Here's how the part is built. I have some questions about the finished solid (model axes, mm). Round coordinates to 2 decimals unless told otherwise and drop trailing zeros. Loops run counter-clockwise (first coordinate to the right, second up) from the corner with the lowest first, then second, coordinate; pieces in that order, holes last. Notation, with made-up numbers: (41, -4.5) - (53, -4.5) arc R21 cw to (53, 32.5) - close; hole circle Ø3 at (22, -6.5). An arc over 180 degrees is marked (long way). Answer as a JSON object with one key per item and string values. Group by question number.
1) I want a section at D-D, the plane x = 110. Please give me the cut outline in (y, z), then the cut area to 3 significant figures.
2) I want a section at A-A, the plane z = -90. Please give me the cut outline in (x, y).
3) Will these pins go through, and if not, where does the flat tip stop? P1, Ø1, axis at x = 47, y = 2, coming from the +Z side; P2, Ø7, axis at x = -110, z = -17.5, coming from the +Y side; P3, Ø10.5, axis at x = 0, z = -127.5, coming from the -Y side.
4) I want a section at B-B, the plane y = 1.65. Please give me the cut outline in (x, z).
5) I want a section at C-C, the plane z = -17.5. Please give me the cut outline in (x, y).
6) If I drill on line 1 along X through (y, z) = (2.95, -80); line 2 along X through (y, z) = (2.95, -17.5); line 3 along Z through (x, y) = (110, 2.85), over which ranges is the centre line in solid material (lowest first)? Write a range as [from, to].
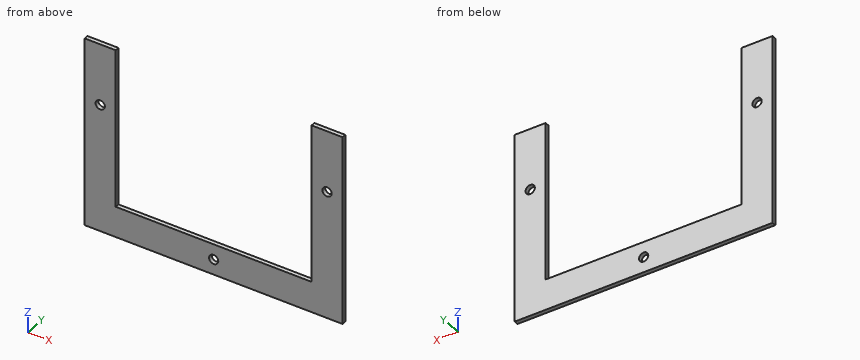
from build123d import *

# Parameters (mm, degrees)
SKETCH1_W            = 250
SKETCH1_H            = 285
SKETCH1_W_2          = 190
SKETCH1_H_2          = 225
EXTRUDE_THIN1_DEPTH  = 4
SKETCH2_W            = 250
SKETCH2_H            = 100
CUT_EXTRUDE1_DEPTH   = 10
SKETCH3_R            = 4.5
CUT_EXTRUDE2_DEPTH   = 10
LPATTERN1_COUNT      = 2
LPATTERN1_PITCH      = 144.5
LPATTERN1_COUNT_DIR2 = 2
LPATTERN1_PITCH_DIR2 = 144.5
SKETCH4_R            = 4.5
CUT_EXTRUDE3_DEPTH   = 10


with BuildPart() as part:
    # Sketch1 → Extrude-Thin1 (new body)
    with BuildSketch(Plane(origin=(0, 0, 0), x_dir=(1, 0, 0), z_dir=(0, 1, 0))):
        Rectangle(SKETCH1_W, SKETCH1_H)
        Rectangle(SKETCH1_W_2, SKETCH1_H_2, mode=Mode.SUBTRACT)
    extrude(amount=EXTRUDE_THIN1_DEPTH)

    # Sketch2 → Cut-Extrude1 (cut)
    with BuildSketch(Plane.XZ):
        with Locations((0, 92.5)):
            Rectangle(SKETCH2_W, SKETCH2_H)
    extrude(amount=-CUT_EXTRUDE1_DEPTH, mode=Mode.SUBTRACT)

    # Sketch3 → Cut-Extrude2 (cut)
    with BuildSketch(Plane.XZ):
        with Locations(Location((0, -127.5, 0), (0, 0, 270))):
            Circle(SKETCH3_R)
    cut_extrude2 = extrude(amount=-CUT_EXTRUDE2_DEPTH, mode=Mode.SUBTRACT)

    # LPattern1: Cut-Extrude2 2 × 2
    with Locations(*[Vector(-1, 0, 0) * (i * LPATTERN1_PITCH) + Vector(-1, 0, 0) * (j * LPATTERN1_PITCH_DIR2) for i in range(LPATTERN1_COUNT) for j in range(LPATTERN1_COUNT_DIR2) if (i, j) != (0, 0)]):
        add(cut_extrude2, mode=Mode.SUBTRACT)

    # Sketch4 → Cut-Extrude3 (cut)
    with BuildSketch(Plane(origin=(0, 0, 0), x_dir=(-1, 0, 0), z_dir=(0, -1, 0))):
        with Locations(Location((110, 17.5, 0), (0, 0, 90))):
            Circle(SKETCH4_R)
    cut_extrude3 = extrude(amount=-CUT_EXTRUDE3_DEPTH, mode=Mode.SUBTRACT)

    # Mirror1: Cut-Extrude3 across plane
    add(cut_extrude3.mirror(Plane(origin=(0, 0, 0), x_dir=(0, 0, 1), z_dir=(1, 0, 0))), mode=Mode.SUBTRACT)


solid = part.part
Outcome:
{
 "1": {"outline": "(0, -142.5) - (4, -142.5) - (4, -22) - (0, -22) - close; (0, -13) - (4, -13) - (4, 42.5) - (0, 42.5) - close", "area": "704 mm^2"},
 "2": {"outline": "(-125, 0) - (-95, 0) - (-95, 4) - (-125, 4) - close; (95, 0) - (125, 0) - (125, 4) - (95, 4) - close"},
 "3": {"P1": "z = -112.5", "P2": "through", "P3": "y = 0"},
 "4": {"outline": "(-125, -142.5) - (125, -142.5) - (125, 42.5) - (95, 42.5) - (95, -112.5) - (-95, -112.5) - (-95, 42.5) - (-125, 42.5) - close; hole circle Ø9 at (-110, -17.5); hole circle Ø9 at (0, -127.5); hole circle Ø9 at (110, -17.5)"},
 "5": {"outline": "(-125, 0) - (-114.5, 0) - (-114.5, 4) - (-125, 4) - close; (-105.5, 0) - (-95, 0) - (-95, 4) - (-105.5, 4) - close; (95, 0) - (105.5, 0) - (105.5, 4) - (95, 4) - close; (114.5, 0) - (125, 0) - (125, 4) - (114.5, 4) - close"},
 "6": {"line 1": "[-125, -95], [95, 125]", "line 2": "[-125, -114.5], [-105.5, -95], [95, 105.5], [114.5, 125]", "line 3": "[-142.5, -22], [-13, 42.5]"}
}
